Input: part model. Units: mm. Frame: model coordinates. A direction names the side the tool comes from. Round coordinates to 2 decimals unless told otherwise and drop trailing zeros. Loops run counter-clockwise (first coordinate to the right, second up) from the corner with the lowest first, then second, coordinate; pieces in that order, holes last. Notation, with made-up numbers: (-24, -30) - (27, -30) arc R19 cw to (27, 6) - close; hole circle Ø4 at (15, 15.5). An arc over 180 degrees is marked (long way). Use CSV: the item, a comma, the result in double quotes. Start each with the question number.
1. Material intervals for probe 1 along Y at (x, z) = (11.5, 2); probe 2 along X at (y, z) = (-40, 5.5) (3 decimals); probe 3 along Z at (x, y) = (-0.5, -20), sorted ascending. Write a range as from..to.
2. Access query for faces 5 (the flat face through (0, -6, 8.7)), 6 (the cylindrical face through (-0.3, -40.87, -7.93)), 7 (the flat face through (-3.175, -42, 6)). Directions: +Z, -Z, +X, -X, +Y, -Y. A direction counts if a zero-diameter tool reaches every point of the face in a straight line with its end or side. Return the directions, or none.
3. Cut plane A-A (z = 0). Return loops of the section in (x, y), and give its area (3 significant figures).
4. Cut plane D-D (x = -9). Return loops of the section in (y, z).
5. Cut plane C-C (y = -21). Return loops of the section in (x, z) (1 decimal), and give its area (3 significant figures).
6. Pin query (flat end, axial travel): P1, Ø2, axis at y = -45.5, z = 5.5, coming from the +X side; P2, Ø9, axis at x = 1.5, y = -5.5, coming from the +Z side; P3, Ø2.5, axis at y = -7.5, z = 10.5, coming from the -X side; P4, Ø1, axis at x = -2.5, z = -2, coming from the +Y side. Return the tip coordinate at first contact, or that it passes through.
7. Pull-direction query (X, two-part tool) for faces 1 (the flat face through (3.175, -42, 6)), 2 (the flat face through (0, -42, 4.762)), 3 (the flat face through (0, 0, 0)), 4 (the cylindrical face through (-0.5, -6.26, -12.69)); classes: +X half, -X half, draft (parallel to the pull), parting line (faces both ways), or undercut.
8. Cut plane B-B (x = 0). Return loops of the section in (y, z), and give its area (3 significant figures).
```python
from build123d import *

# Parameters (mm, degrees)
F0_R     = 12.7
F1_DEPTH = 12.7
F2_R     = 7.9375
F3_DEPTH = 57.15
F4_W     = 8
F4_H     = 8
F5_DEPTH = 69.851
F6_W     = 6.35
F6_H     = 6.35
F7_DEPTH = 57.15


with BuildPart() as f1:
    # F0 (on Front) → F1 (new body)
    with BuildSketch(Plane.XZ):
        Circle(F0_R)
    extrude(amount=F1_DEPTH)

    # F2 (on face) → F3 (join)
    with BuildSketch(Plane.XZ.offset(12.7)):
        Circle(F2_R)
    extrude(amount=F3_DEPTH)

    # F4 (on face) → F5 (cut, through all)
    with BuildSketch(Plane(origin=(0, 0, 0), x_dir=(-1, 0, 0), z_dir=(0, 1, 0))):
        with Locations((0, 12.7)):
            Rectangle(F4_W, F4_H)
    extrude(amount=-F5_DEPTH, mode=Mode.SUBTRACT)

    # F6 (on face) → F7 (cut)
    with BuildSketch(Plane.XZ.offset(69.85)):
        with Locations((0, 7.9375)):
            Rectangle(F6_W, F6_H)
    extrude(amount=-F7_DEPTH, mode=Mode.SUBTRACT)


solid = f1.part
```
Established:
1,probe 1,"y = -12.7..0"
1,probe 2,"x = -5.723..-3.175, 3.175..5.723"
1,probe 3,"z = -7.92..4.76"
2,face 5,"+Z, +Y, -Y"
2,face 6,"-Y"
2,face 7,"+Z, -Y"
3,outline,"(-12.7, -12.7) - (-7.94, -12.7) - (-7.94, -69.85) - (7.94, -69.85) - (7.94, -12.7) - (12.7, -12.7) - (12.7, 0) - (-12.7, 0) - close"
3,area,"1,230 mm2"
4,outline,"(-12.7, -8.96) - (0, -8.96) - (0, 8.96) - (-12.7, 8.96) - close"
5,outline,"(-3.2, 4.8) - (-3.2, 7.3) arc R7.9 ccw (long way) to (3.2, 7.3) - (3.2, 4.8) - close"
5,area,"179 mm2"
6,P1,"stops at x = 6.54"
6,P2,"stops at z = 12.05"
6,P3,"stops at x = -8.7"
6,P4,"stops at y = 0"
7,face 1,"undercut"
7,face 2,"undercut"
7,face 3,"draft"
7,face 4,"parting line"
8,outline,"(-69.85, -7.94) - (-12.7, -7.94) - (-12.7, -12.7) - (0, -12.7) - (0, 8.7) - (-12.7, 8.7) - (-12.7, 4.76) - (-69.85, 4.76) - close"
8,area,"998 mm2"
